```python
from build123d import *

# Parameters (mm, degrees)
F1_DEPTH = 50
F2_W     = 59.939869
F2_H     = 135.170739
F3_DEPTH = 25


with BuildPart() as f1:
    # F0 (on Top) → F1 (new body)
    with BuildSketch(Plane.XY):
        Polygon((37.273418, 19.90559), (-51.23112, -34.814954), (37.273418, -34.814954), align=None)
    extrude(amount=F1_DEPTH)

    # F2 (on Top) → F3 (join)
    with BuildSketch(Plane.XY):
        with Locations((15.658964, -15.171492)):
            Rectangle(F2_W, F2_H)
    extrude(amount=F3_DEPTH)


solid = f1.part
```
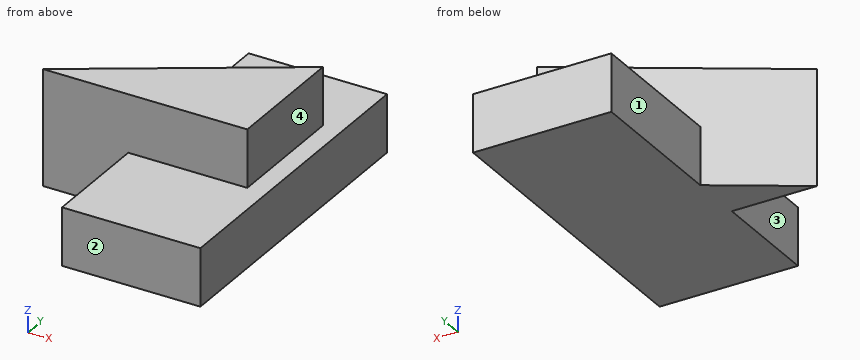
Design review of the part built by this model. Coordinates are the model's own, in mm. Face numbers are marked on the shaded views. A direction names the side the tool comes from. Coordinates: 2 decimals unless noted, no trailing zeros. Loops run counter-clockwise (first coordinate to the right, second up) from the corner with the lowest first, then second, coordinate; pieces in that order, holes last.
Q1. We need section C-C on y = 15. State the section outline as (x, z) points.
Reported:
outline: (-14.31, 0) - (45.63, 0) - (45.63, 25) - (37.27, 25) - (37.27, 50) - (29.34, 50) - (29.34, 25) - (-14.31, 25) - close
Q2. We need section B-B on x = -7. State the section outline as (y, z) points, and give its area (3 significant figures).
Reported:
outline: (-82.76, 0) - (52.41, 0) - (52.41, 25) - (-7.47, 25) - (-7.47, 50) - (-34.81, 50) - (-34.81, 25) - (-82.76, 25) - close
area: 4,060 mm2
Q3. We need section A-A on z = 18. State the section outline as (x, y) points.
Reported:
outline: (-51.23, -34.81) - (-14.31, -34.81) - (-14.31, -82.76) - (45.63, -82.76) - (45.63, 52.41) - (-14.31, 52.41) - (-14.31, -11.99) - close
Q4. To check wall thickness, follow line 1 (Z direction, x = 22, y = -48); line 2 (X direction, y = 13, z = 11); line 3 (Y direction, x = -26.5, z = 14). State the ranges of each line that lie inside material, in increasing order.
Reported:
line 1: z = 0 to 25
line 2: x = -14.31 to 45.63
line 3: y = -34.81 to -19.52
Q5. For pin 1 (5 mm diameter, centred on y = -12, z = 37.5, fed in from +X); pin 2 (7.5 mm diameter, centred on y = -62.5, z = 8, fed in from -X); pin 3 (6 mm diameter, centred on x = -33, z = 12.5, fed in from -Y), all flat-tipped, find the tip position at first contact; note any pin that passes through.
Reported:
pin 1: stops at x = 37.27
pin 2: stops at x = -14.31
pin 3: stops at y = -34.81
Q6. Tool access review of the marked faces 1, 2, 3 and 4: name each direction out of +Z, -Z, +X, -X, +Y, -Y from which nothing blocks a thin tool from reaching the whole face with its end or side.
Reported:
face 1: +Z, -Z, -X, +Y
face 2: +Z, -Z, +X, -X, -Y
face 3: +Z, -Z, -X, -Y
face 4: +Z, +X, +Y, -Y
Q7. We need section D-D on z = 34.5. State the section outline as (x, y) points, and give its area (3 significant figures).
Reported:
outline: (-51.23, -34.81) - (37.27, -34.81) - (37.27, 19.91) - close
area: 2,420 mm2
